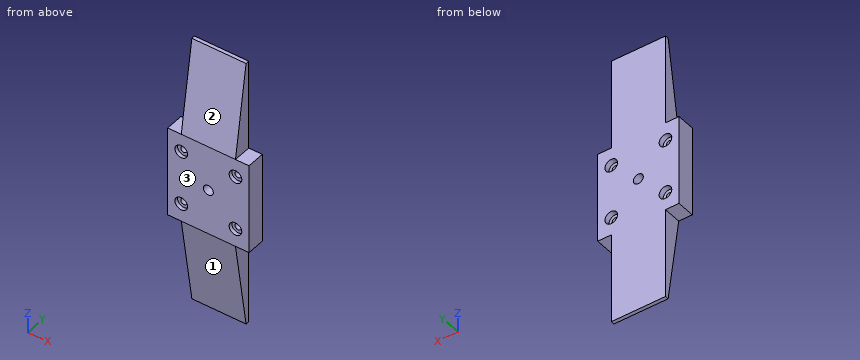
from build123d import *

# Parameters (mm, degrees)
BOSS_EXTRUDE1_DEPTH = 45
SKETCH3_R           = 3.5
CUT_EXTRUDE1_DEPTH  = 2
SKETCH4_R           = 1.75
CUT_EXTRUDE2_DEPTH  = 8
CUT_EXTRUDE3_START  = -3
SKETCH5_R           = 3.5
CUT_EXTRUDE3_DEPTH  = 3
CUT_EXTRUDE4_DEPTH  = 7.5
SKETCH8_R           = 2.75
CUT_EXTRUDE5_DEPTH  = 10


with BuildPart() as part:
    # Sketch2 → Boss-Extrude1 (new body)
    with BuildSketch(Plane(origin=(0, 0, 0), x_dir=(0, 0, -1), z_dir=(1, 0, 0))):
        Polygon((-75, 0), (75, 0), (75, -2), (25, -10), (-25, -10), (-75, -2), align=None)
    extrude(amount=BOSS_EXTRUDE1_DEPTH)

    # Sketch3 → Cut-Extrude1 (cut)
    with BuildSketch(Plane.XZ.offset(10)):
        with Locations(Location((7.5, 15, 0), (0, 0, 270))):
            Circle(SKETCH3_R)
        with Locations(Location((37.5, 15, 0), (0, 0, 270))):
            Circle(SKETCH3_R)
        with Locations(Location((37.5, -15, 0), (0, 0, 270))):
            Circle(SKETCH3_R)
        with Locations(Location((7.5, -15, 0), (0, 0, 270))):
            Circle(SKETCH3_R)
    extrude(amount=-CUT_EXTRUDE1_DEPTH, mode=Mode.SUBTRACT)

    # Sketch4 → Cut-Extrude2 (cut)
    with BuildSketch(Plane.XZ.offset(8)):
        with Locations(Location((7.5, 15, 0), (0, 0, 270))):
            Circle(SKETCH4_R)
        with Locations(Location((7.5, -15, 0), (0, 0, 270))):
            Circle(SKETCH4_R)
        with Locations(Location((37.5, -15, 0), (0, 0, 270))):
            Circle(SKETCH4_R)
        with Locations(Location((37.5, 15, 0), (0, 0, 270))):
            Circle(SKETCH4_R)
    extrude(amount=-CUT_EXTRUDE2_DEPTH, mode=Mode.SUBTRACT)

    # Sketch5 → Cut-Extrude3 (cut)
    with BuildSketch(Plane(origin=(0, 0, 0), x_dir=(1, 0, 0), z_dir=(0, 1, 0)).offset(CUT_EXTRUDE3_START)):
        with Locations(Location((7.5, 15, 0), (0, 0, 90))):
            Circle(SKETCH5_R)
        with Locations(Location((37.5, 15, 0), (0, 0, 90))):
            Circle(SKETCH5_R)
        with Locations(Location((7.5, -15, 0), (0, 0, 90))):
            Circle(SKETCH5_R)
        with Locations(Location((37.5, -15, 0), (0, 0, 90))):
            Circle(SKETCH5_R)
    extrude(amount=CUT_EXTRUDE3_DEPTH, mode=Mode.SUBTRACT)

    # Sketch6 → Cut-Extrude4 (cut)
    with BuildSketch(Plane(origin=(45, 0, 0), x_dir=(0, 0, -1), z_dir=(1, 0, 0))):
        Polygon((25, -10), (25, 0), (75, 0), (75, -2), align=None)
        Polygon((-25, -10), (-25, 0), (-75, 0), (-75, -2), align=None)
    cut_extrude4 = extrude(amount=-CUT_EXTRUDE4_DEPTH, mode=Mode.SUBTRACT)

    # Mirror1: Cut-Extrude4 across plane
    add(cut_extrude4.mirror(Plane(origin=(22.5, 0, 0), x_dir=(0, 0, 1), z_dir=(1, 0, 0))), mode=Mode.SUBTRACT)

    # Sketch8 → Cut-Extrude5 (cut)
    with BuildSketch(Plane.XZ.offset(10)):
        with Locations(Location((22.5, 0, 0), (0, 0, 270))):
            Circle(SKETCH8_R)
    extrude(amount=-CUT_EXTRUDE5_DEPTH, mode=Mode.SUBTRACT)


solid = part.part
Can you work these out from the model? Positions are in its coordinate system, mm. Face numbers are marked on the shaded views. Round coordinates to 2 decimals unless told otherwise and drop trailing zeros. Loops run counter-clockwise (first coordinate to the right, second up) from the corner with the lowest first, then second, coordinate; pieces in that order, holes last. Notation, with made-up numbers: (64, 84.5) - (76, 84.5) arc R31 cw to (76, 123.5) - close; hole circle Ø8 at (-16.5, 87). An arc over 180 degrees is marked (long way). Answer in a Markdown table with one row per item. Add a question column.
Q1. I want a section at B-B on z = 0. List the corners of the cut face in (x, y) for me.
Q2. I want a section at D-D on y = -5.5. List the corners of the cut face in (x, z) for me (3 decimals).
Q3. For pin 1 Ø5 at (y, z) = (-4, 57.5) entering from +X; pin 2 Ø2 at (x, z) = (9, -15) entering from +Y; pin 3 Ø5.5 at (x, z) = (37.5, -14) entering from -Y; pin 4 Ø1.5 at (y, z) = (-3.5, -57) entering from -X, each with a flat end and sliding along its axis, tell me the tip position at first contact or that it passes through.
Q4. I want a section at C-C on z = -15. List the corners of the cut face in (x, y) for me.
Q5. I want a section at A-A on x = 22.5. List the corners of the cut face in (y, z) for me, and give its area (4 significant figures).
Q6. I need wall thicknesses on L1, parallel to X at y = -1.8, z = -15; L2, parallel to X at y = -6.55, z = 15; L3, parallel to X at y = -6, z = 0. Which ranges of each line are inside material? Lowest first, please.
Q7. We'd pull the mould along Z, two halves only. Please class the marked faces 1, 2 and 3: pulls with the +Z half, pulls with the -Z half, needs draft (parallel to the pull), parting line crosses it, or undercut.
A:
| question | item | result |
|---|---|---|
| 1 | outline | (0, -10) - (19.75, -10) - (19.75, 0) - (0, 0) - close; (25.25, -10) - (45, -10) - (45, 0) - (25.25, 0) - close |
| 2 | outline | (0, -25) - (7.5, -25) - (7.5, -53.125) - (37.5, -53.125) - (37.5, -25) - (45, -25) - (45, 25) - (37.5, 25) - (37.5, 53.125) - (7.5, 53.125) - (7.5, 25) - (0, 25) - close; hole circle Ø3.5 at (7.5, -15); hole circle Ø3.5 at (7.5, 15); hole circle Ø5.5 at (22.5, 0); hole circle Ø3.5 at (37.5, -15); hole circle Ø3.5 at (37.5, 15) |
| 3 | pin 1 | x = 37.5 |
| 3 | pin 2 | y = -3 |
| 3 | pin 3 | y = -10 |
| 3 | pin 4 | x = 7.5 |
| 4 | outline | (0, -10) - (4, -10) - (4, -8) - (5.75, -8) - (5.75, -3) - (4, -3) - (4, 0) - (0, 0) - close; (9.25, -8) - (11, -8) - (11, -10) - (34, -10) - (34, -8) - (35.75, -8) - (35.75, -3) - (34, -3) - (34, 0) - (11, 0) - (11, -3) - (9.25, -3) - close; (39.25, -8) - (41, -8) - (41, -10) - (45, -10) - (45, 0) - (41, 0) - (41, -3) - (39.25, -3) - close |
| 5 | outline | (-10, -25) - (-2, -75) - (0, -75) - (0, -2.75) - (-10, -2.75) - close; (-10, 2.75) - (0, 2.75) - (0, 75) - (-2, 75) - (-10, 25) - close |
| 5 | area | 1,045 mm^2 |
| 6 | L1 | 0 to 4, 11 to 34, 41 to 45 |
| 6 | L2 | 0 to 5.75, 9.25 to 35.75, 39.25 to 45 |
| 6 | L3 | 0 to 19.75, 25.25 to 45 |
| 7 | face 1 | pulls with the -Z half |
| 7 | face 2 | pulls with the +Z half |
| 7 | face 3 | needs draft |
